```python
from build123d import *

# Parameters (mm, degrees)
SKIZZE1_W                        = 300
SKIZZE1_H                        = 270
AUFSATZ_LINEAR_AUSTRAGEN1_DEPTH  = 4
F_8_3_8_3_DURCHMESSER_BOHRUNG1_D = 8.3
F_5_1_5_1_DURCHMESSER_BOHRUNG2_D = 5.1
SKIZZE9_W                        = 15
SKIZZE9_H                        = 105
SCHNITT_LINEAR_AUSTRAGEN1_DEPTH  = 11
VERRUNDUNG1_R                    = 3.25
M4_GEWINDEBOHRUNG1_D             = 2.5
SCHNITT_LINEAR_AUSTRAGEN2_DEPTH  = 404.628542103
VERRUNDUNG2_R                    = 1.1
F_5_1_5_1_DURCHMESSER_BOHRUNG1_D = 5.1
SCHNITT_LINEAR_AUSTRAGEN3_REACH  = 405.629
SKIZZE16_R                       = 10.5
SCHNITT_LINEAR_AUSTRAGEN4_REACH  = 405.629
SKIZZE17_R                       = 12
SKIZZE18_R                       = 11.25
SCHNITT_LINEAR_AUSTRAGEN5_DEPTH  = 6.5
SCHNITT_LINEAR_AUSTRAGEN6_DEPTH  = 6
F_2_6_2_6_DURCHMESSER_BOHRUNG1_D = 2.6
SCHNITT_LINEAR_AUSTRAGEN7_REACH  = 405.629
SKIZZE23_R                       = 6.05
M3_GEWINDEBOHRUNG1_D             = 2.5
M3_GEWINDEBOHRUNG1_DEPTH         = 8
M3_GEWINDEBOHRUNG1_TIP           = 0.751075774
M3_GEWINDEBOHRUNG2_D             = 2.5
M3_GEWINDEBOHRUNG2_DEPTH         = 8
M3_GEWINDEBOHRUNG2_TIP           = 0.751075774


with BuildPart() as part:
    # Skizze1 → Aufsatz-Linear austragen1 (new body)
    with BuildSketch(Plane.XY):
        with Locations((150, 135)):
            Rectangle(SKIZZE1_W, SKIZZE1_H)
    extrude(amount=AUFSATZ_LINEAR_AUSTRAGEN1_DEPTH)

    # Ø8.3 (8.3) Durchmesser Bohrung1 (through all)
    with Locations(Plane.XY.offset(4)):
        with Locations((102.5, 15), (172.5, 15), (172.5, 150), (102.5, 150)):
            Hole(F_8_3_8_3_DURCHMESSER_BOHRUNG1_D / 2)

    # Ø5.1 (5.1) Durchmesser Bohrung2 (through all)
    with Locations(Plane(origin=(0, 0, 0), x_dir=(-1, 0, 0), z_dir=(0, 0, -1))):
        with Locations((-235, 252.5), (-87.5, 157.5), (-187.5, 157.5), (-207.5, 252.5)):
            Hole(F_5_1_5_1_DURCHMESSER_BOHRUNG2_D / 2)

    # Skizze9 → Schnitt-Linear austragen1 (cut)
    with BuildSketch(Plane.XY.offset(4)):
        with Locations((137.5, 82.5)):
            Rectangle(SKIZZE9_W, SKIZZE9_H)
    extrude(amount=-SCHNITT_LINEAR_AUSTRAGEN1_DEPTH, mode=Mode.SUBTRACT)

    # Verrundung1
    verrundung1_edges = [part.edges().sort_by_distance(p)[0] for p in [
        (145, 135, 2),
        (145, 30, 2),
        (130, 30, 2),
        (130, 135, 2),
    ]]
    fillet(verrundung1_edges, radius=VERRUNDUNG1_R)

    # M4 Gewindebohrung1 (through all)
    with Locations(Plane(origin=(0, 0, 0), x_dir=(-1, 0, 0), z_dir=(0, 0, -1))):
        with Locations((-158.5, 244), (-116.5, 244)):
            Hole(M4_GEWINDEBOHRUNG1_D / 2)

    # Skizze14 → Schnitt-Linear austragen2 (cut, through all)
    with BuildSketch(Plane.XY.offset(4)):
        with BuildLine():
            Line((234.296375886, 223.828589986), (231.659332685, 222.306092384))
            ThreePointArc((231.659332685, 222.306092384), (232.245330666, 219.070473927), (231.848780407, 215.806217759))
            Line((231.848780407, 215.806217759), (236.275206042, 213.250619727))
            ThreePointArc((236.275206042, 213.250619727), (235.106406461, 210.75), (233.525206042, 208.487480007))
            Line((233.525206042, 208.487480007), (229.098780407, 211.043078039))
            ThreePointArc((229.098780407, 211.043078039), (226.470126771, 209.067527357), (223.375, 207.957207266))
            Line((223.375, 207.957207266), (223.375, 204.912212063))
            ThreePointArc((223.375, 204.912212063), (221.25, 204.75), (219.125, 204.912212063))
            Line((219.125, 204.912212063), (219.125, 207.957207266))
            ThreePointArc((219.125, 207.957207266), (216.029873229, 209.067527357), (213.401219593, 211.043078039))
            Line((213.401219593, 211.043078039), (208.974793958, 208.487480007))
            ThreePointArc((208.974793958, 208.487480007), (207.393593539, 210.75), (206.224793958, 213.250619727))
            Line((206.224793958, 213.250619727), (210.651219593, 215.806217759))
            ThreePointArc((210.651219593, 215.806217759), (210.254669334, 219.070473927), (210.840667315, 222.306092384))
            Line((210.840667315, 222.306092384), (208.203624114, 223.828589986))
            ThreePointArc((208.203624114, 223.828589986), (209.125644347, 225.75), (210.328624114, 227.509197952))
            Line((210.328624114, 227.509197952), (212.965667315, 225.98670035))
            ThreePointArc((212.965667315, 225.98670035), (215.474796105, 228.111998717), (218.5, 229.400704202))
            Line((218.5, 229.400704202), (218.5, 234.511900266))
            ThreePointArc((218.5, 234.511900266), (221.25, 234.75), (224, 234.511900266))
            Line((224, 234.511900266), (224, 229.400704202))
            ThreePointArc((224, 229.400704202), (227.025203895, 228.111998717), (229.534332685, 225.98670035))
            Line((229.534332685, 225.98670035), (232.171375886, 227.509197952))
            ThreePointArc((232.171375886, 227.509197952), (233.374355653, 225.75), (234.296375886, 223.828589986))
        make_face()
    extrude(amount=-SCHNITT_LINEAR_AUSTRAGEN2_DEPTH, mode=Mode.SUBTRACT)

    # Verrundung2
    verrundung2_edges = [part.edges().sort_by_distance(p)[0] for p in [
        (224, 229.400704202, 2),
        (229.534332685, 225.98670035, 2),
        (232.171375886, 227.509197952, 2),
        (234.296375886, 223.828589986, 2),
        (231.659332685, 222.306092384, 2),
        (231.848780407, 215.806217759, 2),
        (236.275206042, 213.250619727, 2),
        (233.525206042, 208.487480007, 2),
        (229.098780407, 211.043078039, 2),
        (223.375, 207.957207266, 2),
        (223.375, 204.912212063, 2),
        (219.125, 204.912212063, 2),
        (219.125, 207.957207266, 2),
        (213.401219593, 211.043078039, 2),
        (208.974793958, 208.487480007, 2),
        (206.224793958, 213.250619727, 2),
        (210.651219593, 215.806217759, 2),
        (210.840667315, 222.306092384, 2),
        (208.203624114, 223.828589986, 2),
        (210.328624114, 227.509197952, 2),
        (212.965667315, 225.98670035, 2),
        (218.5, 229.400704202, 2),
        (218.5, 234.511900266, 2),
        (224, 234.511900266, 2),
    ]]
    fillet(verrundung2_edges, radius=VERRUNDUNG2_R)

    # Ø5.1 (5.1) Durchmesser Bohrung1 (through all)
    with Locations(Plane(origin=(285, 210, 0), x_dir=(-1, 0, 0), z_dir=(0, 0, -1))):
        with Locations((0, 0), (0, -150), (270, 0), (270, -150)):
            Hole(F_5_1_5_1_DURCHMESSER_BOHRUNG1_D / 2)

    # Skizze16 → Schnitt-Linear austragen3 (cut, up to next)
    with BuildSketch(Plane(origin=(0, 0, 0), x_dir=(-1, 0, 0), z_dir=(0, 0, -1)), mode=Mode.PRIVATE) as schnitt_linear_austragen3_sk1:
        with Locations((-261, 134)):
            Circle(SKIZZE16_R)
    schnitt_linear_austragen3_tool1 = extrude(schnitt_linear_austragen3_sk1.sketch, amount=-SCHNITT_LINEAR_AUSTRAGEN3_REACH, mode=Mode.PRIVATE) & part.part
    add(schnitt_linear_austragen3_tool1.solids().sort_by_distance((261, 134, 0))[0], mode=Mode.SUBTRACT)

    # Skizze17 → Schnitt-Linear austragen4 (cut, up to next)
    with BuildSketch(Plane(origin=(0, 0, 0), x_dir=(-1, 0, 0), z_dir=(0, 0, -1)), mode=Mode.PRIVATE) as schnitt_linear_austragen4_sk1:
        with Locations((-261, 168)):
            Circle(SKIZZE17_R)
    schnitt_linear_austragen4_tool1 = extrude(schnitt_linear_austragen4_sk1.sketch, amount=-SCHNITT_LINEAR_AUSTRAGEN4_REACH, mode=Mode.PRIVATE) & part.part
    add(schnitt_linear_austragen4_tool1.solids().sort_by_distance((261, 168, 0))[0], mode=Mode.SUBTRACT)

    # Skizze18 → Schnitt-Linear austragen5 (cut)
    with BuildSketch(Plane.XY.offset(4)):
        with Locations((261, 134)):
            Circle(SKIZZE18_R)
    extrude(amount=-SCHNITT_LINEAR_AUSTRAGEN5_DEPTH, mode=Mode.SUBTRACT)

    # Skizze19 → Schnitt-Linear austragen6 (cut)
    with BuildSketch(Plane.XY.offset(4)):
        with BuildLine():
            Line((248.2, 183), (273.8, 183))
            ThreePointArc((273.8, 183), (275.355634919, 182.355634919), (276, 180.8))
            Line((276, 180.8), (276, 155.2))
            ThreePointArc((276, 155.2), (275.355634919, 153.644365081), (273.8, 153))
            Line((273.8, 153), (248.2, 153))
            ThreePointArc((248.2, 153), (246.644365081, 153.644365081), (246, 155.2))
            Line((246, 155.2), (246, 180.8))
            ThreePointArc((246, 180.8), (246.644365081, 182.355634919), (248.2, 183))
        make_face()
    extrude(amount=-SCHNITT_LINEAR_AUSTRAGEN6_DEPTH, mode=Mode.SUBTRACT)

    # Ø2.6 (2.6) Durchmesser Bohrung1 (through all)
    with Locations(Plane(origin=(0, 0, 0), x_dir=(-1, 0, 0), z_dir=(0, 0, -1))):
        with Locations((-255, 67), (-267, 49)):
            Hole(F_2_6_2_6_DURCHMESSER_BOHRUNG1_D / 2)

    # Skizze23 → Schnitt-Linear austragen7 (cut, up to next)
    with BuildSketch(Plane(origin=(0, 0, 0), x_dir=(-1, 0, 0), z_dir=(0, 0, -1)), mode=Mode.PRIVATE) as schnitt_linear_austragen7_sk1:
        with Locations((-261, 218.75)):
            Circle(SKIZZE23_R)
    schnitt_linear_austragen7_tool1 = extrude(schnitt_linear_austragen7_sk1.sketch, amount=-SCHNITT_LINEAR_AUSTRAGEN7_REACH, mode=Mode.PRIVATE) & part.part
    add(schnitt_linear_austragen7_tool1.solids().sort_by_distance((261, 218.75, 0))[0], mode=Mode.SUBTRACT)

    # M3 Gewindebohrung1
    with Locations(Plane.XY.offset(4)):
        with Locations((250, 151), (272, 151)):
            Hole(M3_GEWINDEBOHRUNG1_D / 2, depth=M3_GEWINDEBOHRUNG1_DEPTH)
            with Locations((0, 0, -(M3_GEWINDEBOHRUNG1_DEPTH + M3_GEWINDEBOHRUNG1_TIP / 2))):  # 118° drill point
                Cone(0, M3_GEWINDEBOHRUNG1_D / 2, M3_GEWINDEBOHRUNG1_TIP, mode=Mode.SUBTRACT)

    # M3 Gewindebohrung2
    with Locations(Plane(origin=(0, 0, 0), x_dir=(-1, 0, 0), z_dir=(0, 0, -1))):
        with Locations((-163.5, 82.5), (-111.5, 82.5)):
            Hole(M3_GEWINDEBOHRUNG2_D / 2, depth=M3_GEWINDEBOHRUNG2_DEPTH)
            with Locations((0, 0, -(M3_GEWINDEBOHRUNG2_DEPTH + M3_GEWINDEBOHRUNG2_TIP / 2))):  # 118° drill point
                Cone(0, M3_GEWINDEBOHRUNG2_D / 2, M3_GEWINDEBOHRUNG2_TIP, mode=Mode.SUBTRACT)


solid = part.part
```
Source: CAD feature listing. Evaluate the final solid. Frame: model axes, mm. Coordinates: 2 decimals unless noted, no trailing zeros. Order: outer loops, then holes, each group sorted by start corner. A loop starts at its lowest first (then second) coordinate and runs counter-clockwise, first axis right, second up. Notation, with made-up numbers: (-8, -1) - (31, -1) arc R14 ccw to (31, 9) - close; hole circle Ø10 at (-3.75, 47.5). An arc over 180 degrees is marked (long way). One line per item, written item: value.
1) Cut plane B-B on y = 76. Output: boundary loops of the cut face in (x, z), plus the area to 3 significant figures.
Computed values:
outline: (0, 0) - (130, 0) - (130, 4) - (0, 4) - close; (145, 0) - (300, 0) - (300, 4) - (145, 4) - close
area: 1,140 mm^2
2) Cut plane C-C on z = 2.8. State how many separate pieces and enclosed holes the cut face has, plus the area to 3 significant figures.
Computed values:
separate pieces: 1
enclosed holes: 25
area: 77,100 mm^2
3) Cut plane A-A on x = 261. Output: boundary loops of the cut face in (y, z).
Computed values:
outline: (0, 0) - (122.75, 0) - (122.75, 4) - (0, 4) - close; (145.25, 0) - (153, 0) - (153, 4) - (145.25, 4) - close; (183, 0) - (212.7, 0) - (212.7, 4) - (183, 4) - close; (224.8, 0) - (270, 0) - (270, 4) - (224.8, 4) - close
4) Contact query for a flat-ended pin moving along its axis: pin 1 (4 mm diameter, centred on x = 267, y = 49, fed in from +Z). Output: stop coordinate, or through.
Computed values:
pin 1: stops at z = 4
5) Ray query, line 1 (X direction, y = 252.5, z = 1.9); line 2 (Y direction, x = 172.5, z = 2.35); line 3 (X direction, y = 82.5, z = 1.7). Return the intervals inside material, ascending. Write a range as [from, to].
Computed values:
line 1: x = [0, 204.95], [210.05, 232.45], [237.55, 300]
line 2: y = [0, 10.85], [19.15, 145.85], [154.15, 270]
line 3: x = [0, 110.25], [112.75, 130], [145, 162.25], [164.75, 300]
